Geometry check sheet. Reference: drawing and pictorial views, mm from the part's lowest x, y, z. A direction names the side the tool comes from. Coordinates: 2 decimals unless noted, no trailing zeros. Write each loop counter-clockwise with the first axis right and the second up, starting at its lowest first coordinate (ties: lowest second). Pieces come first, ordered by that corner, then holes. Notation, with made-up numbers: (44.25, -1) -> (63.25, -1) arc R17 cw to (63.25, 6) -> close; hole circle Ø6 at (32.5, 3). An arc over 180 degrees is marked (long way). Use a Markdown table: item, result. Add a question column.
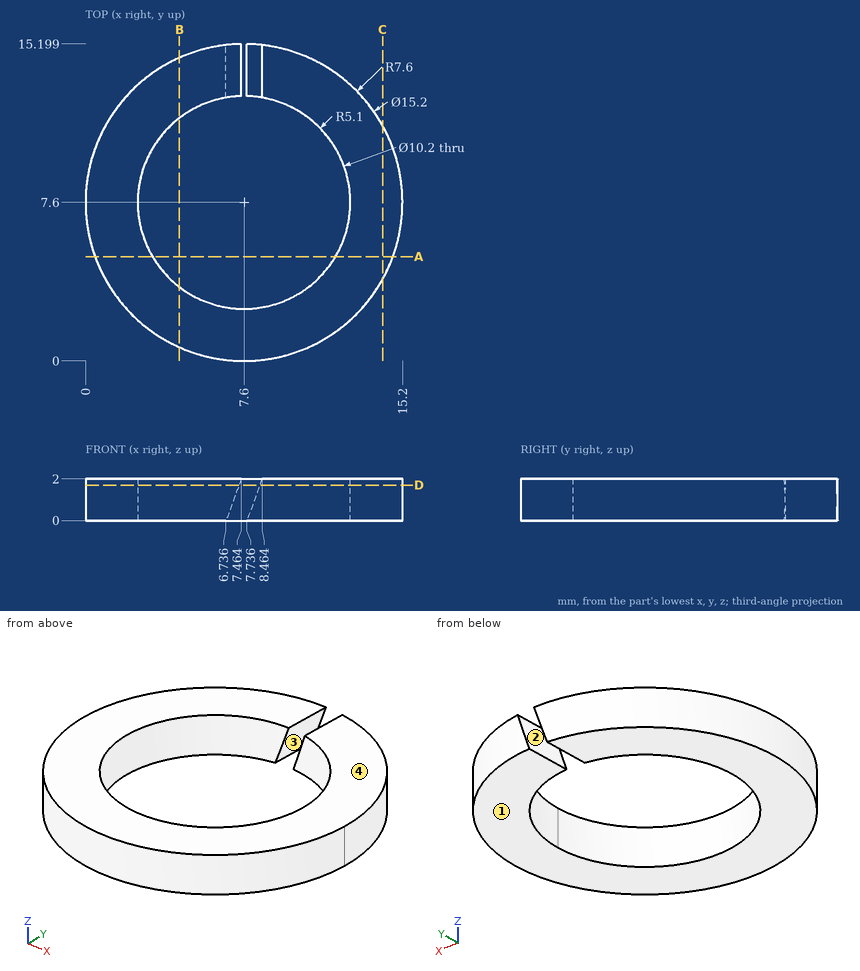
1) Cross-section at C-C on x = 14.25. Record the boundary of the cut face in (y, z).
2) Thickness scan on L1, parallel to X at y = 7.6, z = 1.5; L2, parallel to Y at x = 10.75, z = 1.1; L3, parallel to Y at x = 5.75, z = 0.8. Record the ranges inside material, lowest first.
3) Cross-section at B-B on x = 4.5. Record the boundary of the cut face in (y, z).
4) Set-up check for the marked faces 3 and 4: record each of +Z, -Z, +X, -X, +Y, -Y from which the full face is reachable in a straight line by a thin tool's end or side.
5) Gauge pin test, flat end, axial feed: pin 1 (8 mm diameter, centred on x = 8.5, y = 3.5, fed in from -Z). Record the tip position at first contact, or that the pin passes through.
6) Cross-section at D-D on z = 1.7. Record the boundary of the cut face in (x, y) (1 decimal).
7) Release check for a two-part mould opening along X. For the marked faces 1 and 2 record: released by +X, released by -X, zero draft, split by the parting line, or undercut.
8) Cross-section at A-A on y = 5. Record the boundary of the cut face in (x, z).
Returned:
| question | item | result |
|---|---|---|
| 1 | outline | (3.92, 0) -> (11.28, 0) -> (11.28, 2) -> (3.92, 2) -> close |
| 2 | L1 | x = 0 to 2.5, 12.7 to 15.2 |
| 2 | L2 | y = 0.68 to 3.59, 11.61 to 14.52 |
| 2 | L3 | y = 0.23 to 2.85, 12.35 to 14.97 |
| 3 | outline | (0.66, 0) -> (3.55, 0) -> (3.55, 2) -> (0.66, 2) -> close; (11.65, 0) -> (14.54, 0) -> (14.54, 2) -> (11.65, 2) -> close |
| 4 | face 3 | -Z, +Y |
| 4 | face 4 | +Z, +X, -X, +Y, -Y |
| 5 | pin 1 | stops at z = 0 |
| 6 | outline | (7.4, 12.7) -> (7.4, 15.2) arc R7.6 ccw (long way) to (8.4, 15.2) -> (8.4, 12.6) arc R5.1 cw (long way) to start |
| 7 | face 1 | zero draft |
| 7 | face 2 | undercut |
| 8 | outline | (0.46, 0) -> (3.21, 0) -> (3.21, 2) -> (0.46, 2) -> close; (11.99, 0) -> (14.74, 0) -> (14.74, 2) -> (11.99, 2) -> close |
